The model under review builds one solid part; all positions refer to its coordinate system, in mm. Coordinates: 2 decimals unless noted, no trailing zeros. Loops run counter-clockwise (first coordinate to the right, second up) from the corner with the lowest first, then second, coordinate; pieces in that order, holes last. Notation, with made-up numbers: M -33.5,39 L 4.5,39 A8 ccw 4.5,53 Z; hole C 52,72.25 d11. An arc over 180 degrees is marked long. Use CSV: the item, a comma, the result in double quotes. Start each with the question number.
from build123d import *

# Parameters (mm, degrees)
F0_R     = 2.54
F0_W     = 81.28
F0_H     = 91.44
F0_R_2   = 14.605
F1_DEPTH = 3.175


with BuildPart() as f1:
    # F0 (on Top) → F1 (new body)
    with BuildSketch(Plane.XY):
        with BuildLine():
            ThreePointArc((0, 12.7), (-8.980256, -8.980256), (12.7, 0))
            Line((12.7, 0), (444.5, 0))
            ThreePointArc((444.5, 0), (466.180256, -8.980256), (457.2, 12.7))
            Line((457.2, 12.7), (457.2, 114.3))
            ThreePointArc((457.2, 114.3), (466.180256, 135.980256), (444.5, 127))
            Line((444.5, 127), (12.7, 127))
            ThreePointArc((12.7, 127), (-8.980256, 135.980256), (0, 114.3))
            Line((0, 114.3), (0, 12.7))
        make_face()
        Circle(F0_R, mode=Mode.SUBTRACT)
        with Locations((72.991565, 63.5)):
            Rectangle(F0_W, F0_H, mode=Mode.SUBTRACT)
        with Locations((207.432806, 36.346115)):
            Circle(F0_R_2, mode=Mode.SUBTRACT)
        with Locations((457.2, 0)):
            Circle(F0_R, mode=Mode.SUBTRACT)
        with Locations((309.938095, 43.678654)):
            Circle(F0_R_2, mode=Mode.SUBTRACT)
        with Locations((346.480779, 43.678654)):
            Circle(F0_R_2, mode=Mode.SUBTRACT)
        with Locations((400.783628, 39.574253)):
            Circle(F0_R_2, mode=Mode.SUBTRACT)
        with Locations((170.657456, 63.713811)):
            Circle(F0_R_2, mode=Mode.SUBTRACT)
        with Locations((207.432806, 91.081508)):
            Circle(F0_R_2, mode=Mode.SUBTRACT)
        with Locations((0, 127)):
            Circle(F0_R, mode=Mode.SUBTRACT)
        with Locations((259.465441, 63.713811)):
            Circle(F0_R_2, mode=Mode.SUBTRACT)
        with Locations((309.938095, 85.946283)):
            Circle(F0_R_2, mode=Mode.SUBTRACT)
        with Locations((346.480779, 85.946283)):
            Circle(F0_R_2, mode=Mode.SUBTRACT)
        with Locations((400.783628, 88.493755)):
            Circle(F0_R_2, mode=Mode.SUBTRACT)
        with Locations((457.2, 127)):
            Circle(F0_R, mode=Mode.SUBTRACT)
    extrude(amount=F1_DEPTH)


solid = f1.part
1. Add section D-D (x = 278.5). Write out the cut boundary in (y, z) (3 decimals).
2. Add section A-A (x = 42). Write out the cut boundary in (y, z) (3 decimals).
3. Add section B-B (z = 1.75). Give the number of separate pieces and of enclosed holes in the cut face, plus the area to 3 significant figures.
4. Insertion check: pin 1 Ø1 at (y, z) = (76.5, 2.5) entering from -X; pin 2 Ø1 at (x, z) = (89.5, 1) entering from +Y. Each pin has a flat end and moves straight along its axis. Give the tip position at first contact, or say it passes through.
5. Draft analysis for pull direction X (two halves, no side actions). For faces 1 (the flat face through (225, 65, 3.175)), 2 (the cylindrical face through (414.7, 44, 1.6)), 3 (the cylindrical face through (220.924, 85.488, 1.565)), state which applies: released by +X, released by -X, zero draft, split by the parting line, or undercut.
6. To check wall thickness, follow line 1 along X through (y, z) = (65, 0.85); line 2 along Y through (x, z) = (400, 0.2); line 3 along X through (y, z) = (63.5, 2.2). State the ranges of each line that lie inside material, in increasing order.
7. Add section C-C (x = 164). Write out the cut boundary in (y, z) (3 decimals).
Solved:
1,outline,"M 0,0 L 127,0 L 127,3.175 L 0,3.175 Z"
2,outline,"M 0,0 L 17.78,0 L 17.78,3.175 L 0,3.175 Z; M 109.22,0 L 127,0 L 127,3.175 L 109.22,3.175 Z"
3,separate pieces,"1"
3,enclosed holes,"15"
3,area,"45,400 mm^2"
4,pin 1,"stops at x = 0"
4,pin 2,"stops at y = 127"
5,face 1,"zero draft"
5,face 2,"undercut"
5,face 3,"undercut"
6,line 1,"x = 0 to 32.35, 113.63 to 156.11, 185.21 to 244.92, 274.01 to 457.2"
6,line 2,"y = 0 to 24.99, 54.16 to 73.91, 103.08 to 127"
6,line 3,"x = 0 to 32.35, 113.63 to 156.05, 185.26 to 244.86, 274.07 to 457.2"
7,outline,"M 0,0 L 50.714,0 L 50.714,3.175 L 0,3.175 Z; M 76.713,0 L 127,0 L 127,3.175 L 76.713,3.175 Z"
